```python
from build123d import *

# Parameters (mm, degrees)
SKETCH1_R           = 1.1
BOSS_EXTRUDE1_DEPTH = 1.651
SKETCH2_R           = 1.1
BOSS_EXTRUDE2_DEPTH = 1.651
SKETCH3_R           = 2.1
SKETCH3_R_2         = 1.1
BOSS_EXTRUDE3_DEPTH = 11.811
SKETCH4_W           = 21.082
SKETCH4_H           = 54.737
BOSS_EXTRUDE4_DEPTH = 6.35


with BuildPart() as part:
    # Sketch1 → Boss-Extrude1 (new body)
    with BuildSketch(Plane(origin=(0, 0, 0), x_dir=(1, 0, 0), z_dir=(0, 1, 0))):
        with BuildLine():
            Line((-0.635, -3.175), (32.385, -3.175))
            ThreePointArc((32.385, -3.175), (34.181051224, -2.431051224), (34.925, -0.635))
            Line((34.925, -0.635), (34.925, 45.085))
            ThreePointArc((34.925, 45.085), (34.181051224, 46.881051224), (32.385, 47.625))
            Line((32.385, 47.625), (-0.635, 47.625))
            ThreePointArc((-0.635, 47.625), (-2.431051224, 46.881051224), (-3.175, 45.085))
            Line((-3.175, 45.085), (-3.175, -0.635))
            ThreePointArc((-3.175, -0.635), (-2.431051224, -2.431051224), (-0.635, -3.175))
        make_face()
        with Locations((0, 44.45)):
            Circle(SKETCH1_R, mode=Mode.SUBTRACT)
        with Locations((31.75, 44.45)):
            Circle(SKETCH1_R, mode=Mode.SUBTRACT)
        with Locations((31.75, 0)):
            Circle(SKETCH1_R, mode=Mode.SUBTRACT)
        Circle(SKETCH1_R, mode=Mode.SUBTRACT)
    extrude(amount=BOSS_EXTRUDE1_DEPTH)



with BuildPart() as body_2:
    # Sketch2 → Boss-Extrude2 (new body)
    with BuildSketch(Plane(origin=(0, 15.113, 0), x_dir=(-1, 0, 0), z_dir=(0, -1, 0))):
        with BuildLine():
            Line((3.175, -0.635), (3.175, 45.085))
            ThreePointArc((3.175, 45.085), (2.431051224, 46.881051224), (0.635, 47.625))
            Line((0.635, 47.625), (-32.385, 47.625))
            ThreePointArc((-32.385, 47.625), (-34.181051224, 46.881051224), (-34.925, 45.085))
            Line((-34.925, 45.085), (-34.925, -0.635))
            ThreePointArc((-34.925, -0.635), (-34.181051224, -2.431051224), (-32.385, -3.175))
            Line((-32.385, -3.175), (0.635, -3.175))
            ThreePointArc((0.635, -3.175), (2.431051224, -2.431051224), (3.175, -0.635))
        make_face()
        with Locations((-31.75, 44.45)):
            Circle(SKETCH2_R, mode=Mode.SUBTRACT)
        with Locations((0, 44.45)):
            Circle(SKETCH2_R, mode=Mode.SUBTRACT)
        with Locations((-31.75, 0)):
            Circle(SKETCH2_R, mode=Mode.SUBTRACT)
        Circle(SKETCH2_R, mode=Mode.SUBTRACT)
    extrude(amount=BOSS_EXTRUDE2_DEPTH)


with BuildPart() as part_1:
    add(part.part)

    add(body_2.part)  # Boss-Extrude3 merges body 2
    # Sketch3 → Boss-Extrude3 (add)
    with BuildSketch(Plane(origin=(0, 1.651, 0), x_dir=(1, 0, 0), z_dir=(0, 1, 0))):
        Circle(SKETCH3_R)
        Circle(SKETCH3_R_2, mode=Mode.SUBTRACT)
        with Locations((31.75, 0)):
            Circle(SKETCH3_R)
        with Locations((31.75, 0)):
            Circle(SKETCH3_R_2, mode=Mode.SUBTRACT)
        with Locations((31.75, 44.45)):
            Circle(SKETCH3_R)
        with Locations((31.75, 44.45)):
            Circle(SKETCH3_R_2, mode=Mode.SUBTRACT)
        with Locations((0, 44.45)):
            Circle(SKETCH3_R)
        with Locations((0, 44.45)):
            Circle(SKETCH3_R_2, mode=Mode.SUBTRACT)
    extrude(amount=BOSS_EXTRUDE3_DEPTH)

    # Sketch4 → Boss-Extrude4 (add)
    with BuildSketch(Plane(origin=(0, 15.113, 0), x_dir=(1, 0, 0), z_dir=(0, 1, 0))):
        with Locations((15.875, 20.2565)):
            Rectangle(SKETCH4_W, SKETCH4_H)
    extrude(amount=BOSS_EXTRUDE4_DEPTH)


solid = part_1.part
```
The model under review builds one solid part; all positions refer to its coordinate system, in mm. A direction names the side the tool comes from. Coordinates: 2 decimals unless noted, no trailing zeros. Write each loop counter-clockwise with the first axis right and the second up, starting at its lowest first coordinate (ties: lowest second). Pieces come first, ordered by that corner, then holes. Notation, with made-up numbers: (-36, 43) -> (-18, 43) arc R32 cw to (-18, 77) -> close; hole circle Ø2 at (72, 8.5). An arc over 180 degrees is marked (long way). One line per item, written item: value. Start each with the question number.
Q1. For faces 4 (the face through (16, 1, 3.175)), 5 (the face through (31.3, 7.5, -42.4)), 6 (the face through (-2.45, 14.3, -46.86)), 7 (the face through (31, 15.113, -23)), 8 (the face through (-2.45, 0.81, 2.41)), list the 3-axis set-ups (+Z, -Z, +X, -X, +Y, -Y) from which the entire face can be reached by the end or side of a thin tool; tool diameter is ignored.
Q2. Add section B-B, the plane z = 0. Give the boundary of the cut face in (x, y) (3 decimals), then the cut area to 3 significant figures.
Q3. The part is to be moulded in two halves that separate along Y. For faces 1 (the face through (16, 15.113, 5)), 2 (the face through (16, 17, -47.625)), 3 (the face through (29.65, 7.47, -0.09)), say which applies: +Y half, -Y half, draft (parallel to the pull), parting line (faces both ways), or undercut.
Q4. Clearance check with flat-ended pins moving along their axes: P1, Ø5, axis at x = 13, y = 2.5, coming from the +Z side (3 decimals); P2, Ø2.5, axis at x = 31.5, z = -21, coming from the +Y side; P3, Ø1.9, axis at y = 19.5, z = -10.5, coming from the +X side. State where each tip first meets the part, or that it passes through.
Q5. To check wall thickness, follow probe 1 along Z at (x, y) = (31.75, 6.25); probe 2 along X at (y, z) = (4.5, 0); probe 3 along Y at (x, z) = (5.5, -4). State the ranges of each line that lie inside material, in increasing order.
Q6. Add section A-A, the plane y = 12.5. Give the boundary of the cut face in (x, z), then the cut area to 3 significant figures.
Q7. Add section D-D, the plane x = 7. Give the boundary of the cut face in (y, z) (3 decimals).
Q8. Add section C-C, the plane x = 31.75. Give the boundary of the cut face in (y, z) (3 decimals), then the cut area to 3 significant figures.
Response:
1. face 4: +Z, +X, -X, -Y
1. face 5: none
1. face 6: -Z, -X, +Y, -Y
1. face 7: +Z, -Z, +X, +Y
1. face 8: +Z, -X, +Y, -Y
2. outline: (-3.175, 0) -> (-1.1, 0) -> (-1.1, 15.113) -> (-3.175, 15.113) -> (-3.175, 13.462) -> (-2.1, 13.462) -> (-2.1, 1.651) -> (-3.175, 1.651) -> close; (1.1, 0) -> (30.65, 0) -> (30.65, 15.113) -> (26.416, 15.113) -> (26.416, 21.463) -> (5.334, 21.463) -> (5.334, 15.113) -> (1.1, 15.113) -> close; (32.85, 0) -> (34.925, 0) -> (34.925, 1.651) -> (33.85, 1.651) -> (33.85, 13.462) -> (34.925, 13.462) -> (34.925, 15.113) -> (32.85, 15.113) -> close; hole (2.1, 1.651) -> (29.65, 1.651) -> (29.65, 13.462) -> (2.1, 13.462) -> close
2. area: 292 mm²
3. face 1: -Y half
3. face 2: draft
3. face 3: undercut
4. P1: z = 3.175
4. P2: y = 15.11
4. P3: x = 26.42
5. probe 1: -46.55 to -45.55, -43.35 to -42.35, -2.1 to -1.1, 1.1 to 2.1
5. probe 2: -2.1 to -1.1, 1.1 to 2.1, 29.65 to 30.65, 32.85 to 33.85
5. probe 3: 0 to 1.65, 13.46 to 21.46
6. outline: circle Ø4.2 at (0, -44.45); circle Ø4.2 at (0, 0); circle Ø4.2 at (31.75, -44.45); circle Ø4.2 at (31.75, 0); hole circle Ø2.2 at (0, -44.45); hole circle Ø2.2 at (0, 0); hole circle Ø2.2 at (31.75, -44.45); hole circle Ø2.2 at (31.75, 0)
6. area: 40.2 mm²
7. outline: (0, -47.625) -> (1.651, -47.625) -> (1.651, 3.175) -> (0, 3.175) -> close; (13.462, -47.625) -> (21.463, -47.625) -> (21.463, 7.112) -> (15.113, 7.112) -> (15.113, 3.175) -> (13.462, 3.175) -> close
8. outline: (0, -47.625) -> (1.651, -47.625) -> (1.651, -46.55) -> (13.462, -46.55) -> (13.462, -47.625) -> (15.113, -47.625) -> (15.113, -45.55) -> (0, -45.55) -> close; (0, -43.35) -> (15.113, -43.35) -> (15.113, -1.1) -> (0, -1.1) -> close; (0, 1.1) -> (15.113, 1.1) -> (15.113, 3.175) -> (13.462, 3.175) -> (13.462, 2.1) -> (1.651, 2.1) -> (1.651, 3.175) -> (0, 3.175) -> close; hole (1.651, -42.35) -> (13.462, -42.35) -> (13.462, -2.1) -> (1.651, -2.1) -> close
8. area: 200 mm²
